Answer from the drawing. Dimensions are ordinates in mm from the lowest x, y and z of the part. Round coordinates to 2 decimals unless told otherwise and drop trailing zeros. Write each loop counter-clockwise with the first axis right and the second up, starting at its lowest first coordinate (ties: lowest second). Pieces come first, ordered by that corner, then holes. Notation, with made-up numbers: (22.5, 59) - (53.5, 59) arc R21 cw to (53.5, 76) - close; hole circle Ø6 at (10, 10). An arc over 180 degrees is marked (long way). One line per item, written item: value. Start each with the question number.
(1) A cutting plane is placed at B-B, the plane z = 152.4. Determine the outline of the cut face in (x, y), plus the area to 3 significant figures.
(2) A cutting plane is placed at A-A, the plane x = 304.8. Determine the outline of the cut face in (y, z).
(3) A cutting plane is placed at C-C, the plane z = 244. Determine the outline of the cut face in (x, y), plus the area to 3 significant figures.
(4) Find the intervals of material crossed by L1, parallel to X at y = 3, z = 393.7; L2, parallel to X at y = 3, z = 264; L3, parallel to Z at x = 321, y = 1, in increasing order.
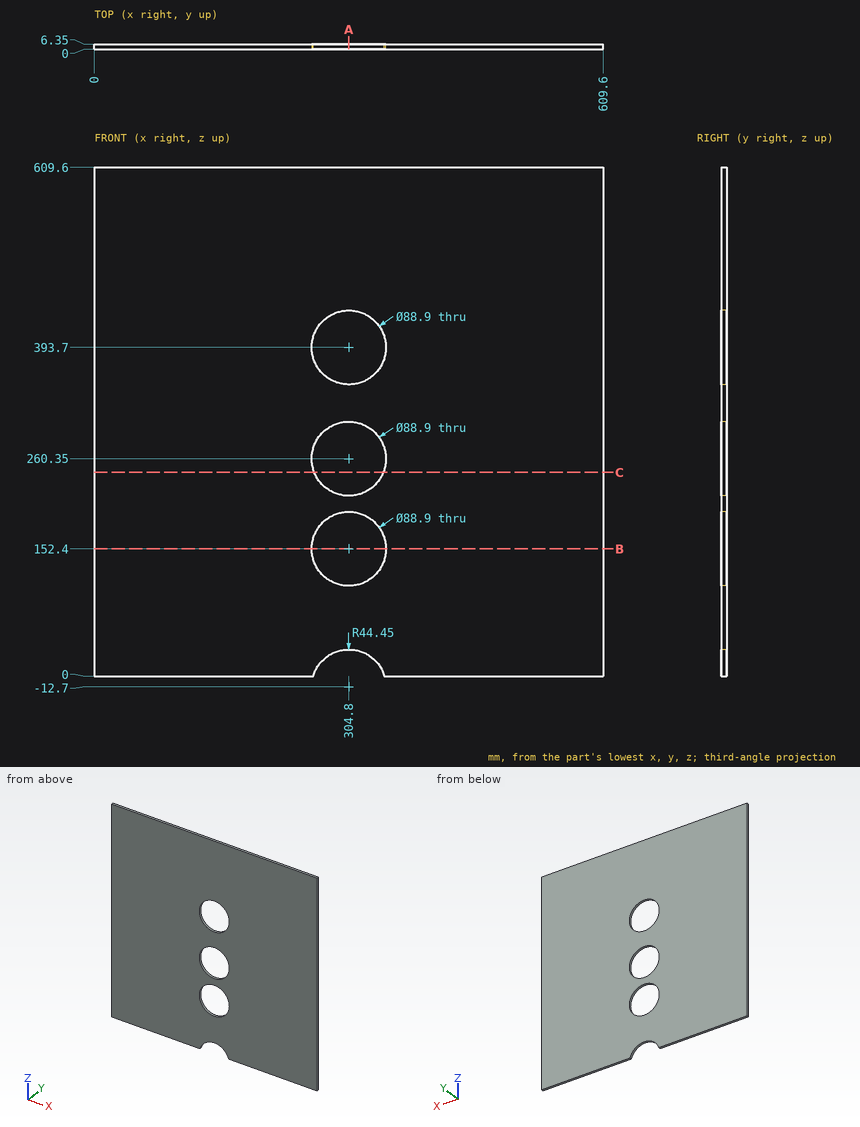
Here are the results:
1. outline: (0, 0) - (260.35, 0) - (260.35, 6.35) - (0, 6.35) - close; (349.25, 0) - (609.6, 0) - (609.6, 6.35) - (349.25, 6.35) - close
1. area: 3,310 mm²
2. outline: (0, 31.75) - (6.35, 31.75) - (6.35, 107.95) - (0, 107.95) - close; (0, 196.85) - (6.35, 196.85) - (6.35, 215.9) - (0, 215.9) - close; (0, 304.8) - (6.35, 304.8) - (6.35, 349.25) - (0, 349.25) - close; (0, 438.15) - (6.35, 438.15) - (6.35, 609.6) - (0, 609.6) - close
3. outline: (0, 0) - (263.47, 0) - (263.47, 6.35) - (0, 6.35) - close; (346.13, 0) - (609.6, 0) - (609.6, 6.35) - (346.13, 6.35) - close
3. area: 3,350 mm²
4. L1: 0 to 260.35, 349.25 to 609.6
4. L2: 0 to 260.5, 349.1 to 609.6
4. L3: 28.69 to 111.01, 193.79 to 218.96, 301.74 to 352.31, 435.09 to 609.6
